from build123d import *

# Parameters (mm, degrees)
SKETCH067_R     = 4
PAD037_DEPTH    = 7
SKETCH068_R     = 6.5
PAD038_DEPTH    = 0.5
SKETCH070_R     = 6.5
PAD039_DEPTH    = 0.5
SKETCH071_R     = 1.5
POCKET037_DEPTH = 8.001


with BuildPart() as part:
    # Sketch067 → Pad037 (new body)
    with BuildSketch(Plane.XY):
        Circle(SKETCH067_R)
    extrude(amount=PAD037_DEPTH)

    # Sketch068 (on Face3 of Pad037) → Pad038 (join)
    with BuildSketch(Plane.XY.offset(7)):
        Circle(SKETCH068_R)
    extrude(amount=PAD038_DEPTH)

    # Sketch070 (on Face5 of Pad038) → Pad039 (join)
    with BuildSketch(Plane(origin=(0, 0, 0), x_dir=(1, 0, 0), z_dir=(0, 0, -1))):
        Circle(SKETCH070_R)
    extrude(amount=PAD039_DEPTH)

    # Sketch071 (on Face3 of Pad039) → Pocket037 (cut, through all)
    with BuildSketch(Plane(origin=(0, 0, -0.5), x_dir=(1, 0, 0), z_dir=(0, 0, -1))):
        Circle(SKETCH071_R)
    extrude(amount=-POCKET037_DEPTH, mode=Mode.SUBTRACT)


solid = part.part
The listing builds one solid part. Answer for the finished solid, in the listing's coordinates (mm). A direction names the side the tool comes from. Round coordinates to 2 decimals unless told otherwise and drop trailing zeros. Order: outer loops, then holes, each group sorted by start corner. A loop starts at its lowest first (then second) coordinate and runs counter-clockwise, first axis right, second up. Notation, with made-up numbers: (-40, -9) -> (1, -9) arc R19 cw to (1, 4) -> close; hole circle Ø5 at (-34, -40). An arc over 180 degrees is marked (long way). Put each result on its own line as item: value.
Q1. Section A-A, the plane y = 0 is taken. Write down the section's boundary in (x, z), and give its area (3 significant figures).
Results list:
outline: (-6.5, -0.5) -> (-1.5, -0.5) -> (-1.5, 7.5) -> (-6.5, 7.5) -> (-6.5, 7) -> (-4, 7) -> (-4, 0) -> (-6.5, 0) -> close; (1.5, -0.5) -> (6.5, -0.5) -> (6.5, 0) -> (4, 0) -> (4, 7) -> (6.5, 7) -> (6.5, 7.5) -> (1.5, 7.5) -> close
area: 45.0 mm^2
Q2. Each of these flat-tipped pins is pushed along its axis until it touches: P1, Ø1, axis at x = -0.5, z = 4.5, coming from the -Y side; P2, Ø2, axis at x = -5, y = -4.5, coming from the -Z side; P3, Ø2.5, axis at x = 0, y = 0, coming from the -Z side; P4, Ø2, axis at y = 2.5, z = 3.5, coming from the +X side. Where does it stop, or does it pass through?
Results list:
P1: y = -4
P2: z = -0.5
P3: through
P4: x = 3.71
Q3. Section D-D, the plane z = 4.25 is taken. Write down the section's boundary in (x, y).
Results list:
outline: circle Ø8 at (0, 0); hole circle Ø3 at (0, 0)
Q4. Consider line 1 along Y through (x, z) = (0, 1.5); line 2 along Z through (x, y) = (3.5, -2.25); line 3 along X through (y, z) = (0.25, 3.25). Determine where each line is inside the solid, lowest interval first.
Results list:
line 1: -4 to -1.5, 1.5 to 4
line 2: -0.5 to 0, 7 to 7.5
line 3: -3.99 to -1.48, 1.48 to 3.99
Q5. Section C-C, the plane x = 2.25 is taken. Write down the section's boundary in (y, z), and give its area (3 significant figures).
Results list:
outline: (-6.1, -0.5) -> (6.1, -0.5) -> (6.1, 0) -> (3.31, 0) -> (3.31, 7) -> (6.1, 7) -> (6.1, 7.5) -> (-6.1, 7.5) -> (-6.1, 7) -> (-3.31, 7) -> (-3.31, 0) -> (-6.1, 0) -> close
area: 58.5 mm^2
Q6. Determine the mould class of faces 3 (the flat face through (0, 2, 7.5)), 4 (the cylindrical face through (-0.867, -3.905, 3.451)), 5 (the cylindrical face through (-1.5, -0.07, 3.44)) for opening direction Y: pulls with the +Y half, pulls with the -Y half, needs draft (parallel to the pull), parting line crosses it, or undercut.
Results list:
face 3: needs draft
face 4: parting line crosses it
face 5: undercut
Q7. Which of the six approach directions +Z, -Z, +X, -X, +Y, -Y give full straight-line access (tool end or side, diameter ignored) to faces 1 (the flat face through (3, -3, 0)), 2 (the flat face through (0, -2, -0.5))?
Results list:
face 1: none
face 2: -Z, +X, -X, +Y, -Y
